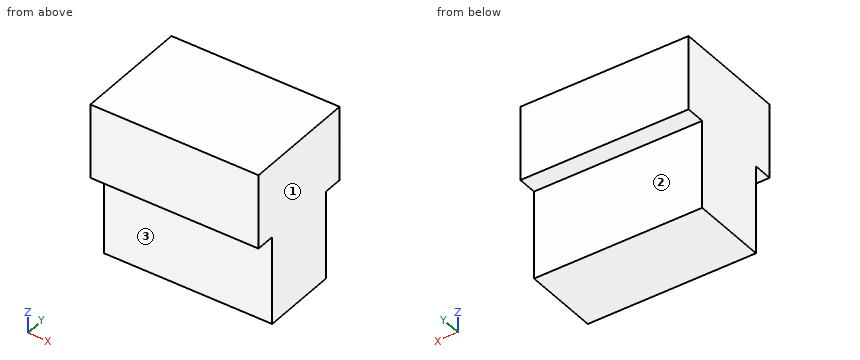
from build123d import *

# Parameters (mm, degrees)
F0_W      = 119.803108
F0_H      = 54.300458
F1_DEPTH  = 32.96413
F1_FACE_W = 119.803108
F1_FACE_H = 54.300458
F2_DEPTH  = 30.10031
F3_W      = 119.803108
F3_H      = 81.823676
F4_DEPTH  = 53.18567


with BuildPart() as f1:
    # F0 (on Top) → F1 (new body)
    with BuildSketch(Plane.XY):
        Rectangle(F0_W, F0_H)
    extrude(amount=F1_DEPTH)

    # F1_face (on face) → F2 (join)
    with BuildSketch(Plane(origin=(0, 0, 0), x_dir=(1, 0, 0), z_dir=(0, 0, -1))):
        Rectangle(F1_FACE_W, F1_FACE_H)
    extrude(amount=F2_DEPTH)

    # F3 (on face) → F4 (join)
    with BuildSketch(Plane.XY.offset(32.96413)):
        Rectangle(F3_W, F3_H)
    extrude(amount=F4_DEPTH)


solid = f1.part
Design review of the part built by this model. Coordinates are the model's own, in mm. Face numbers are marked on the shaded views. A direction names the side the tool comes from. Coordinates: 2 decimals unless noted, no trailing zeros. Order: outer loops, then holes, each group sorted by start corner. A loop starts at its lowest first (then second) coordinate and runs counter-clockwise, first axis right, second up.
Item 1: Take a section at C-C, the plane z = -23. Write out the cut boundary in (x, y), then the cut area to 3 significant figures.
Item 2: Take a section at A-A, the plane x = 0.5. Write out the cut boundary in (y, z).
Item 3: For the marked faces 1, 2 and 3, list the 3-axis set-ups (+Z, -Z, +X, -X, +Y, -Y) from which the entire face can be reached by the end or side of a thin tool; tool diameter is ignored.
Item 4: For line 1 (Z direction, x = 29.5, y = 30); line 2 (Y direction, x = -48.5, z = 32), list the stretches that pass through material, from the lowest coordinate up.
Item 5: For pin 1 Ø1.5 at (x, z) = (-45.5, -8.5) entering from -Y; pin 2 Ø7 at (x, y) = (-25, -33.5) entering from -Z, all flat-tipped, find the tip position at first contact; note any pin that passes through.
Item 6: Take a section at B-B, the plane y = -36. Write out the cut boundary in (x, z).
The answers:
1. outline: (-59.9, -27.15) - (59.9, -27.15) - (59.9, 27.15) - (-59.9, 27.15) - close
1. area: 6,510 mm2
2. outline: (-40.91, 32.96) - (-27.15, 32.96) - (-27.15, -30.1) - (27.15, -30.1) - (27.15, 32.96) - (40.91, 32.96) - (40.91, 86.15) - (-40.91, 86.15) - close
3. face 1: +Z, -Z, +X, +Y, -Y
3. face 2: -Z, +X, -X, +Y
3. face 3: -Z, +X, -X, -Y
4. line 1: z = 32.96 to 86.15
4. line 2: y = -27.15 to 27.15
5. pin 1: stops at y = -27.15
5. pin 2: stops at z = 32.96
6. outline: (-59.9, 32.96) - (59.9, 32.96) - (59.9, 86.15) - (-59.9, 86.15) - close
